For this review, take the finished solid that the model builds, in its own axes (mm). Round coordinates to 2 decimals unless told otherwise and drop trailing zeros. Loops run counter-clockwise (first coordinate to the right, second up) from the corner with the lowest first, then second, coordinate; pieces in that order, holes last.
1. To check wall thickness, follow line 1 along X through (y, z) = (1.75, 75); line 2 along X through (y, z) = (0.4, 76); line 3 along Z through (x, y) = (-12.5, 0.3). State the ranges of each line that lie inside material, in increasing order.
2. Consider section B-B on z = 75. State the section outline as (x, y) points.
3. Consider section A-A on x = -75. State the section outline as (y, z) points.
4. Consider section D-D on z = 47. State the section outline as (x, y) points, then the cut area to 3 significant figures.
5. Consider section C-C on y = 2.8. State the section outline as (x, z) points.
6. Clearance check with a flat-ended pin moving along its axis: pin 1 Ø10 at (x, z) = (-15, 75) entering from +Y. State where the tip first meets the part, or that it passes through.
7. Draft analysis for pull direction X (two halves, no side actions). For faces 1 (the flat face through (-15, 2, 0)), 2 (the cylindrical face through (-14.069, 1.972, 77.957)), 3 (the cylindrical face through (-18.026, 1.972, 14.328)), 4 (the flat face through (-60, 2, 30)), state which applies: released by +X, released by -X, zero draft, split by the parting line, or undercut.
from build123d import *

# Parameters (mm, degrees)
SKETCH1_R           = 3.1
BOSS_EXTRUDE1_DEPTH = 4


with BuildPart() as part:
    # Sketch1 → Boss-Extrude1 (new body)
    with BuildSketch(Plane(origin=(0, 0, 0), x_dir=(1, 0, 0), z_dir=(0, 1, 0))):
        Polygon((0, 0), (0, -90), (-90, -90), (-90, -60), (-30, 0), align=None)
        with Locations(Location((-15, -15, 0), (0, 0, 270))):
            Circle(SKETCH1_R, mode=Mode.SUBTRACT)
        with Locations(Location((-15, -45, 0), (0, 0, 270))):
            Circle(SKETCH1_R, mode=Mode.SUBTRACT)
        with Locations(Location((-15, -75, 0), (0, 0, 270))):
            Circle(SKETCH1_R, mode=Mode.SUBTRACT)
        with Locations(Location((-45, -75, 0), (0, 0, 270))):
            Circle(SKETCH1_R, mode=Mode.SUBTRACT)
        with Locations(Location((-75, -75, 0), (0, 0, 270))):
            Circle(SKETCH1_R, mode=Mode.SUBTRACT)
    extrude(amount=BOSS_EXTRUDE1_DEPTH)


solid = part.part
Resolved:
1. line 1: x = -90 to -78.1, -71.9 to -48.1, -41.9 to -18.1, -11.9 to 0
1. line 2: x = -90 to -77.93, -72.07 to -47.93, -42.07 to -17.93, -12.07 to 0
1. line 3: z = 0 to 13.17, 16.83 to 43.17, 46.83 to 73.17, 76.83 to 90
2. outline: (-90, 0) - (-78.1, 0) - (-78.1, 4) - (-90, 4) - close; (-71.9, 0) - (-48.1, 0) - (-48.1, 4) - (-71.9, 4) - close; (-41.9, 0) - (-18.1, 0) - (-18.1, 4) - (-41.9, 4) - close; (-11.9, 0) - (0, 0) - (0, 4) - (-11.9, 4) - close
3. outline: (0, 45) - (4, 45) - (4, 71.9) - (0, 71.9) - close; (0, 78.1) - (4, 78.1) - (4, 90) - (0, 90) - close
4. outline: (-77, 0) - (-17.37, 0) - (-17.37, 4) - (-77, 4) - close; (-12.63, 0) - (0, 0) - (0, 4) - (-12.63, 4) - close
4. area: 289 mm2
5. outline: (-90, 60) - (-30, 0) - (0, 0) - (0, 90) - (-90, 90) - close; hole circle Ø6.2 at (-75, 75); hole circle Ø6.2 at (-45, 75); hole circle Ø6.2 at (-15, 15); hole circle Ø6.2 at (-15, 45); hole circle Ø6.2 at (-15, 75)
6. pin 1: stops at y = 4
7. face 1: zero draft
7. face 2: undercut
7. face 3: undercut
7. face 4: released by -X
